Check sheet for the modelled part. Datum: model origin and axes. Units: mm. Face numbers are marked on the shaded views. A direction names the side the tool comes from. Give positions to 0.01 mm unless a question says otherwise; leave off trailing zeros. Write each loop counter-clockwise with the first axis right and the second up, starting at its lowest first coordinate (ties: lowest second). Pieces come first, ordered by that corner, then holes. Notation, with made-up numbers: (81, 59) -> (85, 59) arc R30 ccw to (85, 93) -> close; hole circle Ø3 at (-32.75, 27). An arc over 180 degrees is marked (long way). Return JSON: item names as keys, results as strings.
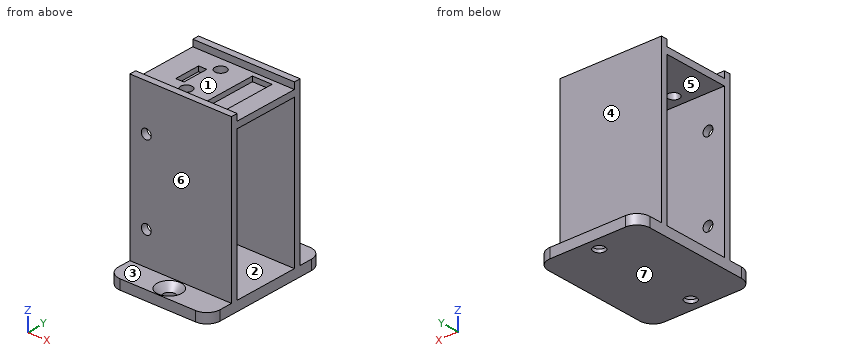
from build123d import *

# Parameters (mm, degrees)
SKETCH1_W           = 31
SKETCH1_H           = 24
BOSS_EXTRUDE1_DEPTH = 2
SKETCH2_W           = 31
SKETCH2_H           = 2
BOSS_EXTRUDE2_DEPTH = 2
SKETCH4_R           = 1.75
CUT_EXTRUDE1_DEPTH  = 3
SKETCH5_W           = 2.5
SKETCH5_H           = 8
SKETCH5_W_2         = 6
SKETCH5_H_2         = 17
CUT_EXTRUDE2_DEPTH  = 1.5
SKETCH6_W           = 31
SKETCH6_H           = 2
BOSS_EXTRUDE4_DEPTH = 48
BOSS_EXTRUDE5_START = 8
SKETCH8_W           = 31
SKETCH8_H           = 3
BOSS_EXTRUDE5_DEPTH = 40
SKETCH9_R           = 1.75
CUT_EXTRUDE3_DEPTH  = 38
CHAMFER1_SIZE       = 2
FILLET1_R           = 4
SKETCH10_R          = 1.5
CUT_EXTRUDE4_DEPTH  = 5


with BuildPart() as part:
    # Sketch1 → Boss-Extrude1 (new body)
    with BuildSketch(Plane.XY):
        with Locations((15.5, 12)):
            Rectangle(SKETCH1_W, SKETCH1_H)
    extrude(amount=BOSS_EXTRUDE1_DEPTH)

    # Sketch2 → Boss-Extrude2 (add)
    with BuildSketch(Plane.XY.offset(2)):
        with Locations((15.5, 23)):
            Rectangle(SKETCH2_W, SKETCH2_H)
        with Locations((15.5, 1)):
            Rectangle(SKETCH2_W, SKETCH2_H)
    extrude(amount=BOSS_EXTRUDE2_DEPTH)

    # Sketch4 → Cut-Extrude1 (cut)
    with BuildSketch(Plane.XY.offset(2)):
        with Locations((12, 18)):
            Circle(SKETCH4_R)
        with Locations((12, 6)):
            Circle(SKETCH4_R)
    extrude(amount=-CUT_EXTRUDE1_DEPTH, mode=Mode.SUBTRACT)

    # Sketch5 → Cut-Extrude2 (cut)
    with BuildSketch(Plane.XY.offset(2)):
        with Locations((8.25, 12)):
            Rectangle(SKETCH5_W, SKETCH5_H)
        with Locations((22.5, 12)):
            Rectangle(SKETCH5_W_2, SKETCH5_H_2)
    extrude(amount=-CUT_EXTRUDE2_DEPTH, mode=Mode.SUBTRACT)

    # Sketch6 → Boss-Extrude4 (add)
    with BuildSketch(Plane(origin=(0, 0, 0), x_dir=(-1, 0, 0), z_dir=(0, 0, -1))):
        with Locations((-15.5, 23)):
            Rectangle(SKETCH6_W, SKETCH6_H)
        with Locations((-15.5, 1)):
            Rectangle(SKETCH6_W, SKETCH6_H)
    extrude(amount=BOSS_EXTRUDE4_DEPTH)

    # Sketch8 → Boss-Extrude5 (add)
    with BuildSketch(Plane.XZ.offset(BOSS_EXTRUDE5_START)):
        with Locations((15.5, -46.5)):
            Rectangle(SKETCH8_W, SKETCH8_H)
    extrude(amount=-BOSS_EXTRUDE5_DEPTH)

    # Sketch9 → Cut-Extrude3 (cut)
    with BuildSketch(Plane.XY.offset(-45)):
        with Locations((15.5, 28)):
            Circle(SKETCH9_R)
        with Locations((15.5, -4)):
            Circle(SKETCH9_R)
    extrude(amount=-CUT_EXTRUDE3_DEPTH, mode=Mode.SUBTRACT)

    # Chamfer1
    chamfer1_edges = [part.edges().sort_by_distance(p)[0] for p in [
        (13.75, 28, -45),
        (13.75, -4, -45),
    ]]
    chamfer(chamfer1_edges, length=CHAMFER1_SIZE)

    # Fillet1
    fillet1_edges = [part.edges().sort_by_distance(p)[0] for p in [
        (0, 32, -46.5),
        (31, 32, -46.5),
        (0, -8, -46.5),
        (31, -8, -46.5),
    ]]
    fillet(fillet1_edges, radius=FILLET1_R)

    # Sketch10 → Cut-Extrude4 (cut)
    with BuildSketch(Plane.XZ):
        with Locations(Location((5, -10, 0), (0, 0, 270))):
            Circle(SKETCH10_R)
        with Locations(Location((5, -35, 0), (0, 0, 270))):
            Circle(SKETCH10_R)
    extrude(amount=-CUT_EXTRUDE4_DEPTH, mode=Mode.SUBTRACT)


solid = part.part
(1) Cross-section at C-C on x = 5. Enter the section's corners in (y, z), then the cut area to 3 significant figures.
Reply:
{"outline": "(-8, -48) -> (32, -48) -> (32, -45) -> (24, -45) -> (24, 4) -> (22, 4) -> (22, 2) -> (2, 2) -> (2, 4) -> (0, 4) -> (0, -8.5) -> (2, -8.5) -> (2, 0) -> (22, 0) -> (22, -45) -> (2, -45) -> (2, -36.5) -> (0, -36.5) -> (0, -45) -> (-8, -45) -> close; (0, -33.5) -> (2, -33.5) -> (2, -11.5) -> (0, -11.5) -> close", "area": "344 mm^2"}
(2) Depth check by flat-ended pin: pin 1 Ø0.8 at (x, z) = (23.5, 1.5) entering from +Y; pin 2 Ø9.5 at (x, z) = (11.5, -16) entering from -Y; pin 3 Ø4 at (x, y) = (15, 27.5) entering from +Z. Enter the tip coordinate at first touch or a pass-through.
Reply:
{"pin 1": "y = 24", "pin 2": "y = 0", "pin 3": "z = -46.04"}
(3) Release check for a two-part mould opening along Y. For the marked faces 4, 5, 6 and 7 record: pulls with the +Y half, pulls with the -Y half, needs draft (parallel to the pull), parting line crosses it, or undercut.
Reply:
{"face 4": "pulls with the +Y half", "face 5": "undercut", "face 6": "pulls with the -Y half", "face 7": "needs draft"}
(4) Cross-section at A-A on z = -21.5. Enter the section's corners in (x, y).
Reply:
{"outline": "(0, 0) -> (31, 0) -> (31, 2) -> (0, 2) -> close; (0, 22) -> (31, 22) -> (31, 24) -> (0, 24) -> close"}
(5) Cross-section at D-D on y = 12. Enter the section's corners in (x, z).
Reply:
{"outline": "(0, -48) -> (31, -48) -> (31, -45) -> (0, -45) -> close; (0, 0) -> (31, 0) -> (31, 2) -> (25.5, 2) -> (25.5, 0.5) -> (19.5, 0.5) -> (19.5, 2) -> (9.5, 2) -> (9.5, 0.5) -> (7, 0.5) -> (7, 2) -> (0, 2) -> close"}
(6) Cross-section at B-B on y = 6. Enter the section's corners in (x, z), then the cut area to 3 significant figures.
Reply:
{"outline": "(0, -48) -> (31, -48) -> (31, -45) -> (0, -45) -> close; (0, 0) -> (10.25, 0) -> (10.25, 2) -> (0, 2) -> close; (13.75, 0) -> (31, 0) -> (31, 2) -> (25.5, 2) -> (25.5, 0.5) -> (19.5, 0.5) -> (19.5, 2) -> (13.75, 2) -> close", "area": "139 mm^2"}
(7) Set-up check for the marked faces 1, 2 and 3: record each of +Z, -Z, +X, -X, +Y, -Y from which the full face is reachable in a straight line by a thin tool's end or side.
Reply:
{"face 1": "+Z, +X, -X", "face 2": "+X, -X", "face 3": "+Z, +X, -X, -Y"}
(8) Thickness scan on L1, parallel to Y at x = 15.5, z = -47.6; L2, parallel to Y at x = 24.5, z = -27; L3, parallel to Z at x = 28, y = 16.5. Record the ranges inside material, lowest first.
Reply:
{"L1": "-8 to -5.75, -2.25 to 26.25, 29.75 to 32", "L2": "0 to 2, 22 to 24", "L3": "-48 to -45, 0 to 2"}
